Work out the finished part from the listing and answer in its coordinate system (mm). Face numbers are marked on the shaded views. Coordinates: 2 decimals unless noted, no trailing zeros. Order: outer loops, then holes, each group sorted by start corner. A loop starts at its lowest first (then second) coordinate and runs counter-clockwise, first axis right, second up. Notation, with made-up numbers: (53.5, 54.25) - (77.5, 54.25) arc R28 cw to (77.5, 88.25) - close; hole circle Ø10 at (-1.5, -18.5). An arc over 180 degrees is marked (long way). Answer as a JSON object with one key per item and string values. Group by question number.
1) Section C-C (x = -103) is taken. Give the vertices of the cut face in (y, z).
2) Section B-B (y = 36) is taken. Give the vertices of the cut face in (x, z), plus the area to 3 significant figures.
3) Section A-A (z = -162) is taken. Give the vertices of the cut face in (x, y), plus the area to 3 significant figures.
4) The mould has two halves that part along Z. Classify the marked faces 1 and 2: released by +Z, released by -Z, zero draft, split by the parting line, or undercut.
5) Each of these flat-tipped pins is pushed along its axis until it touches: P1, Ø4, axis at x = -87, z = 139, coming from the +Y side; P2, Ø11.5, axis at x = 210.5, z = -34, coming from the +Y side. Where does it stop, or does it pass through?
6) Find the intervals of material crossed by line 1 along Y through (x, z) = (-211, -209); line 2 along X through (y, z) = (87, 13.5); line 3 along Y through (x, z) = (-196, 55.5), in increasing order.
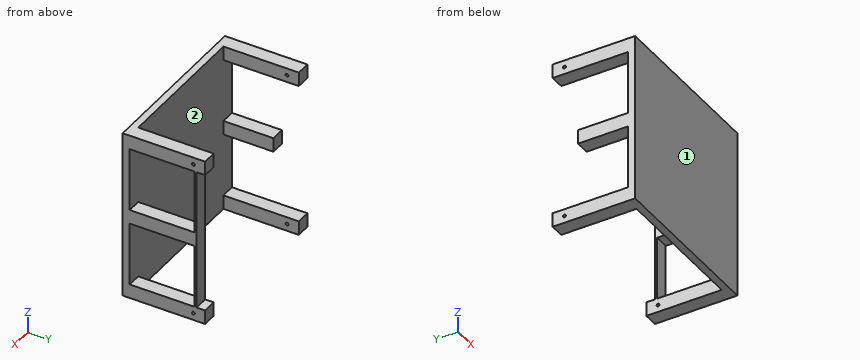
from build123d import *

# Parameters (mm, degrees)
SKETCH2_W           = 457.2
SKETCH2_H           = 457.2
BOSS_EXTRUDE1_DEPTH = 19.05
SKETCH3_W           = 38.1
SKETCH3_H           = 38.1
BOSS_EXTRUDE2_DEPTH = 203.2
SKETCH4_R           = 4
CUT_EXTRUDE1_DEPTH  = 457.2
SKETCH6_W           = 38.1
SKETCH6_H           = 38.1
BOSS_EXTRUDE3_DEPTH = 134.874
SKETCH7_W           = 38.1
SKETCH7_H           = 38.1
BOSS_EXTRUDE4_DEPTH = 173.99
SKETCH8_W           = 38.1
SKETCH8_H           = 381
BOSS_EXTRUDE5_DEPTH = 6.35


with BuildPart() as part:
    # Sketch2 → Boss-Extrude1 (new body)
    with BuildSketch(Plane(origin=(0, 0, 0), x_dir=(1, 0, 0), z_dir=(0, 1, 0))):
        Rectangle(SKETCH2_W, SKETCH2_H)
    extrude(amount=BOSS_EXTRUDE1_DEPTH)

    # Sketch3 → Boss-Extrude2 (add)
    with BuildSketch(Plane(origin=(0, 19.05, 0), x_dir=(1, 0, 0), z_dir=(0, 1, 0))):
        with Locations((209.55, 209.55)):
            Rectangle(SKETCH3_W, SKETCH3_H)
        with Locations((-209.55, 209.55)):
            Rectangle(SKETCH3_W, SKETCH3_H)
        with Locations((-209.55, -209.55)):
            Rectangle(SKETCH3_W, SKETCH3_H)
        with Locations((209.55, -209.55)):
            Rectangle(SKETCH3_W, SKETCH3_H)
    extrude(amount=BOSS_EXTRUDE2_DEPTH)

    # Sketch4 → Cut-Extrude1 (cut)
    with BuildSketch(Plane.ZY.offset(228.6)):
        with Locations((-209.55, 190.5)):
            Circle(SKETCH4_R)
        with Locations(Location((209.55, 190.5, 0), (0, 0, 180))):
            Circle(SKETCH4_R)
    extrude(amount=-CUT_EXTRUDE1_DEPTH, mode=Mode.SUBTRACT)

    # Sketch6 → Boss-Extrude3 (add)
    with BuildSketch(Plane(origin=(0, 19.05, 0), x_dir=(1, 0, 0), z_dir=(0, 1, 0))):
        with Locations((-209.55, 0)):
            Rectangle(SKETCH6_W, SKETCH6_H)
    extrude(amount=BOSS_EXTRUDE3_DEPTH)

    # Sketch7 → Boss-Extrude4 (add)
    with BuildSketch(Plane(origin=(0, 19.05, 0), x_dir=(1, 0, 0), z_dir=(0, 1, 0))):
        with Locations((209.55, 0)):
            Rectangle(SKETCH7_W, SKETCH7_H)
    extrude(amount=BOSS_EXTRUDE4_DEPTH)

    # Sketch8 → Boss-Extrude5 (add)
    with BuildSketch(Plane(origin=(0, 193.04, 0), x_dir=(1, 0, 0), z_dir=(0, 1, 0))):
        with Locations((209.55, 0)):
            Rectangle(SKETCH8_W, SKETCH8_H)
    extrude(amount=BOSS_EXTRUDE5_DEPTH)


solid = part.part
Report:
{
 "1": {"outline": "(0, -228.6) - (19.05, -228.6) - (19.05, 228.6) - (0, 228.6) - close"},
 "2": {"outline": "(-228.6, -228.6) - (-190.5, -228.6) - (-190.5, -190.5) - (-228.6, -190.5) - close; (-228.6, -19.05) - (-190.5, -19.05) - (-190.5, 19.05) - (-228.6, 19.05) - close; (-228.6, 190.5) - (-190.5, 190.5) - (-190.5, 228.6) - (-228.6, 228.6) - close; (190.5, -228.6) - (228.6, -228.6) - (228.6, -190.5) - (190.5, -190.5) - close; (190.5, -19.05) - (228.6, -19.05) - (228.6, 19.05) - (190.5, 19.05) - close; (190.5, 190.5) - (228.6, 190.5) - (228.6, 228.6) - (190.5, 228.6) - close", "area": "8,710 mm²"},
 "3": {"outline": "(-228.6, 0) - (228.6, 0) - (228.6, 19.05) - (-228.6, 19.05) - close; (190.5, 193.04) - (228.6, 193.04) - (228.6, 199.39) - (190.5, 199.39) - close", "area": "8,950 mm²"},
 "4": {"face 1": "zero draft", "face 2": "undercut"},
 "5": {"P1": "stops at y = 19.05", "P2": "stops at y = 199.39"},
 "6": {"line 1": "y = 0 to 186.54, 194.46 to 222.25", "line 2": "x = -228.6 to -190.5, 190.5 to 228.6", "line 3": "y = 0 to 19.05"}
}
